Model file for the job. Use its own axes, mm. Face numbers are marked on the shaded views. A direction names the side the tool comes from. Coordinates: 2 decimals unless noted, no trailing zeros. Order: outer loops, then holes, each group sorted by start corner. A loop starts at its lowest first (then second) coordinate and runs counter-clockwise, first axis right, second up. Notation, with made-up numbers: (73.25, -2.5) -> (92.25, -2.5) arc R23 ccw to (92.25, 19.5) -> close; hole circle Ø11 at (10, 85.5). An arc over 180 degrees is marked (long way). Use CSV: the item, a comma, the result in double quotes. Start each with the question number.
(1) Cut at B-B on z = -35. Write the cut outline in (x, y), plus the area to 3 significant figures.
(2) Probe L1, parallel to Z at x = -39, y = -15; L2, parallel to Z at x = 7, y = -28; L3, parallel to Z at x = 7.5, y = -15. List the from-to ranges inside material, lowest first.
(3) Pull direction Z, two halves, no side cores. Call the marked faces 4, 5 and 6: pulls with the +Z half, pulls with the -Z half, needs draft (parallel to the pull), parting line crosses it, or undercut.
(4) Tool access for the marked faces 1, 2 and 3: list every direction of +Z, -Z, +X, -X, +Y, -Y with a clear straight run to the whole face (end or side of a thin tool).
(5) Cut at A-A on x = 33. Give the number of separate pieces and of enclosed holes in the cut face, plus the area to 3 significant figures.
(6) Cut at D-D on z = -246. Write the cut outline in (x, y).
(7) Pin check, flat tips, straight feed: pin 1 Ø1.5 at (x, y) = (31, 2) entering from +Z; pin 2 Ø12 at (x, z) = (30, -214) entering from -Y; pin 3 Ø1.5 at (x, z) = (-13.5, -211) entering from +Y. Stop position of each tip, or through.
```python
from build123d import *

# Parameters (mm, degrees)
IZIM1_R                      = 17
Y_KSEKLIK_EKSTR_ZYON1_DEPTH  = 25
IZIM2_R                      = 19
Y_KSEKLIK_EKSTR_ZYON2_DEPTH  = 8
Y_KSEKLIK_EKSTR_ZYON3_DEPTH  = 15
IZIM4_R                      = 17
Y_KSEKLIK_EKSTR_ZYON4_DEPTH  = 30
Y_KSEKLIK_EKSTR_ZYON5_DEPTH  = 15
IZIM6_R                      = 17
Y_KSEKLIK_EKSTR_ZYON6_DEPTH  = 5
Y_KSEKLIK_EKSTR_ZYON7_DEPTH  = 15
IZIM9_R                      = 17
Y_KSEKLIK_EKSTR_ZYON8_DEPTH  = 30
Y_KSEKLIK_EKSTR_ZYON9_DEPTH  = 15
IZIM12_R                     = 17
Y_KSEKLIK_EKSTR_ZYON10_DEPTH = 3


with BuildPart() as part:
    # Çizim1 → Yükseklik-Ekstrüzyon1 (new body)
    with BuildSketch(Plane.XY):
        Circle(IZIM1_R)
    extrude(amount=Y_KSEKLIK_EKSTR_ZYON1_DEPTH)

    # Çizim2 → Yükseklik-Ekstrüzyon2 (add)
    with BuildSketch(Plane(origin=(0, 0, 0), x_dir=(-1, 0, 0), z_dir=(0, 0, -1))):
        Circle(IZIM2_R)
    extrude(amount=-Y_KSEKLIK_EKSTR_ZYON2_DEPTH)

    # Çizim3 → Yükseklik-Ekstrüzyon3 (add)
    with BuildSketch(Plane(origin=(0, 0, 0), x_dir=(-1, 0, 0), z_dir=(0, 0, -1))):
        with BuildLine():
            ThreePointArc((-44.415603771, -7.228702626), (-2.027811095, -44.954287695), (43.584396229, -11.198232242))
            ThreePointArc((43.584396229, -11.198232242), (33.112866367, 17.436067755), (13.682042331, 40.931155566))
            ThreePointArc((13.682042331, 40.931155566), (0.405418694, 45.996086199), (-13.05683546, 41.447463263))
            ThreePointArc((-13.05683546, 41.447463263), (-32.757662874, 19.700124785), (-44.415603771, -7.228702626))
        make_face()
    extrude(amount=Y_KSEKLIK_EKSTR_ZYON3_DEPTH)

    # Çizim4 → Yükseklik-Ekstrüzyon4 (add)
    with BuildSketch(Plane(origin=(0, 0, -15), x_dir=(-1, 0, 0), z_dir=(0, 0, -1))):
        with Locations((0, 25)):
            Circle(IZIM4_R)
    extrude(amount=Y_KSEKLIK_EKSTR_ZYON4_DEPTH)

    # Çizim5 → Yükseklik-Ekstrüzyon5 (add)
    with BuildSketch(Plane(origin=(0, 0, -45), x_dir=(-1, 0, 0), z_dir=(0, 0, -1))):
        with BuildLine():
            ThreePointArc((45, 0), (0, 45), (-45, 0))
            ThreePointArc((-45, 0), (-31.68561215, -23.649975334), (-11.926296118, -42.255449988))
            ThreePointArc((-11.926296118, -42.255449988), (0, -45.97067458), (11.926296118, -42.255449988))
            ThreePointArc((11.926296118, -42.255449988), (31.68561215, -23.649975334), (45, 0))
        make_face()
    extrude(amount=Y_KSEKLIK_EKSTR_ZYON5_DEPTH)

    # Çizim6 → Yükseklik-Ekstrüzyon6 (add)
    with BuildSketch(Plane(origin=(0, 0, -60), x_dir=(-1, 0, 0), z_dir=(0, 0, -1))):
        Circle(IZIM6_R)
    extrude(amount=Y_KSEKLIK_EKSTR_ZYON6_DEPTH)

    # Çizim7 → Yükseklik-Ekstrüzyon7 (add)
    with BuildSketch(Plane(origin=(0, 0, -65), x_dir=(-1, 0, 0), z_dir=(0, 0, -1))):
        with BuildLine():
            ThreePointArc((44.457488298, 6.966472151), (2.243897169, 44.944019908), (-43.542511702, 11.360003287))
            ThreePointArc((-43.542511702, 11.360003287), (-32.842453707, -16.531076412), (-14.546498608, -40.145936031))
            ThreePointArc((-14.546498608, -40.145936031), (1.83841745, -45.919374304), (16.965213719, -37.376652353))
            ThreePointArc((16.965213719, -37.376652353), (33.480341406, -16.921835259), (44.457488298, 6.966472151))
        make_face()
    extrude(amount=Y_KSEKLIK_EKSTR_ZYON7_DEPTH)

    # Çizim9 → Yükseklik-Ekstrüzyon8 (add)
    with BuildSketch(Plane(origin=(0, 0, -80), x_dir=(-1, 0, 0), z_dir=(0, 0, -1))):
        with Locations((0, -25)):
            Circle(IZIM9_R)
    extrude(amount=Y_KSEKLIK_EKSTR_ZYON8_DEPTH)

    # Çizim10 → Yükseklik-Ekstrüzyon9 (add)
    with BuildSketch(Plane(origin=(0, 0, -110), x_dir=(-1, 0, 0), z_dir=(0, 0, -1))):
        with BuildLine():
            ThreePointArc((-44.415603771, -7.228702626), (-2.027811095, -44.954287695), (43.584396229, -11.198232242))
            ThreePointArc((43.584396229, -11.198232242), (33.112866367, 17.436067755), (13.682042331, 40.931155566))
            ThreePointArc((13.682042331, 40.931155566), (0.405418694, 45.996086199), (-13.05683546, 41.447463263))
            ThreePointArc((-13.05683546, 41.447463263), (-32.757662874, 19.700124785), (-44.415603771, -7.228702626))
        make_face()
    extrude(amount=Y_KSEKLIK_EKSTR_ZYON9_DEPTH)

    # Çizim12 → Yükseklik-Ekstrüzyon10 (add)
    with BuildSketch(Plane(origin=(0, 0, -125), x_dir=(-1, 0, 0), z_dir=(0, 0, -1))):
        Circle(IZIM12_R)
    extrude(amount=Y_KSEKLIK_EKSTR_ZYON10_DEPTH)

    # Aynalama1: part across plane


with BuildPart() as part_1:
    add(part.part)
    add(part.part.mirror(Plane(origin=(0, 0, -128), x_dir=(1, 0, 0), z_dir=(0, 0, -1))))


solid = part_1.part
```
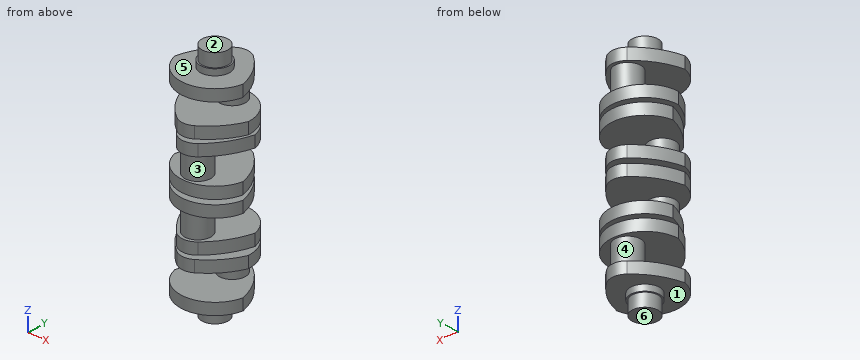
Outcome:
1,outline,"circle Ø34 at (0, 25)"
1,area,"908 mm2"
2,L1,"-256 to -241, -146 to -131, -125 to -110, -15 to 0"
2,L2,"-256 to -241, -211 to -196, -191 to -131, -125 to -65, -60 to -45, -15 to 0"
2,L3,"-281 to -241, -211 to -45, -15 to 25"
3,face 4,"undercut"
3,face 5,"pulls with the +Z half"
3,face 6,"pulls with the -Z half"
4,face 1,"-Z"
4,face 2,"+Z, +X, -X, +Y, -Y"
4,face 3,"none"
5,separate pieces,"8"
5,enclosed holes,"0"
5,area,"5,980 mm2"
6,outline,"(-43.58, -11.2) arc R45 ccw to (44.42, -7.23) arc R90 ccw to (13.06, 41.45) arc R21 ccw to (-13.68, 40.93) arc R90 ccw to start"
7,pin 1,"z = 0"
7,pin 2,"y = -31.46"
7,pin 3,"y = 43.16"
